```python
from build123d import *

# Parameters (mm, degrees)
SKETCH001_R  = 0.965047
PAD_DEPTH    = 4
SKETCH_W     = 14.86762
SKETCH_H     = 20
PAD001_DEPTH = 5


with BuildPart() as part:
    # Sketch001 → Pad (new body)
    with BuildSketch(Plane.XY):
        with BuildLine():
            ThreePointArc((-5, -17.500002), (0, -22.500002), (5, -17.500002))
            Line((5, -17.500002), (5, 0))
            Line((5, 0), (5, 17.500002))
            ThreePointArc((5, 17.500002), (-2e-06, 22.499991), (-5, 17.499998))
            Line((-5, -17.500002), (-5, 17.499998))
        make_face()
        with Locations((0, 17.499991)):
            Circle(SKETCH001_R, mode=Mode.SUBTRACT)
        with Locations((0, -17.500002)):
            Circle(SKETCH001_R, mode=Mode.SUBTRACT)
    extrude(amount=PAD_DEPTH)

    # Sketch (on Face7 of Pad) → Pad001 (join)
    with BuildSketch(Plane.XY.offset(4)):
        with Locations((0.040686, 0)):
            Rectangle(SKETCH_W, SKETCH_H)
    extrude(amount=-PAD001_DEPTH)


solid = part.part
```
Part model, mm, in its own coordinate system. A direction names the side the tool comes from. Round coordinates to 2 decimals unless told otherwise and drop trailing zeros. Loops run counter-clockwise (first coordinate to the right, second up) from the corner with the lowest first, then second, coordinate; pieces in that order, holes last. Notation, with made-up numbers: (-15.5, 39.25) -> (18.5, 39.25) arc R20 cw to (18.5, 64.25) -> close; hole circle Ø3 at (44, 75). An arc over 180 degrees is marked (long way). Use CSV: the item, a comma, the result in double quotes. Start each with the question number.
1) Cut at A-A, the plane z = 2.8. Write the cut outline in (x, y), plus the area to 3 significant figures.
2) Which spindle directions (+Z, -Z, +X, -X, +Y, -Y) get a long thin tool onto all of the face, cutting with end or side? Do faces 4 (the flat face through (-5, 14, 2)), 5 (the flat face through (5, 14, 2)), 6 (the flat face through (-5, -14, 2)), 7 (the flat face through (5, -14, 2)), 8 (the flat face through (0, 16, 0)). Say none if no direction does.
3) Cut at D-D, the plane x = 2.25. Write the cut outline in (y, z).
4) Cut at B-B, the plane x = 0. Write the cut outline in (y, z).
5) Pull direction Y, two halves, no side cores. Call faces 1 (the cylindrical face through (-0.126, -16.543, 1.972)), 2 (the flat face through (7.474, 0, 2)), 3 (the cylindrical face through (-0.1, -22.5, 2)): +Y half, -Y half, draft (parallel to the pull), parting line (faces both ways), or undercut.
6) Drop flat-ended pins along their axis: P1, Ø1.7, axis at x = 0, y = -17.5, coming from the -Z side; P2, Ø8, axis at x = 1.5, y = 18, coming from the -Z side; P3, Ø1, axis at y = 11.5, z = 3, coming from the +X side; P4, Ø2, axis at x = 2.5, z = 0, coming from the +Y side. Give the stop position or say it passes through.
7) Wall check: L1, parallel to Y at x = 0, z = 1.25; L2, parallel to X at y = -11, z = 1.4; L3, parallel to Z at x = -2.5, y = -11.5. Give the ranges that are in metal, low to high. Write a range as [from, to].
8) Cut at C-C, the plane y = -11.5. Write the cut outline in (x, z).
Determined:
1,outline,"(-7.39, -10) -> (-5, -10) -> (-5, -17.5) arc R5 ccw to (5, -17.5) -> (5, -10) -> (7.47, -10) -> (7.47, 10) -> (5, 10) -> (5, 17.5) arc R5 ccw to (-5, 17.5) -> (-5, 10) -> (-7.39, 10) -> close; hole circle Ø1.93 at (0, -17.5); hole circle Ø1.93 at (0, 17.5)"
1,area,"520 mm2"
2,face 4,"+Z, -Z, -X, +Y"
2,face 5,"+Z, -Z, +X, +Y"
2,face 6,"+Z, -Z, -X, -Y"
2,face 7,"+Z, -Z, +X, -Y"
2,face 8,"-Z, +X, -X, +Y"
3,outline,"(-21.97, 0) -> (-10, 0) -> (-10, -1) -> (10, -1) -> (10, 0) -> (21.97, 0) -> (21.97, 4) -> (-21.97, 4) -> close"
4,outline,"(-22.5, 0) -> (-18.47, 0) -> (-18.47, 4) -> (-22.5, 4) -> close; (-16.53, 0) -> (-10, 0) -> (-10, -1) -> (10, -1) -> (10, 0) -> (16.53, 0) -> (16.53, 4) -> (-16.53, 4) -> close; (18.47, 0) -> (22.5, 0) -> (22.5, 4) -> (18.47, 4) -> close"
5,face 1,"undercut"
5,face 2,"draft"
5,face 3,"-Y half"
6,P1,"passes through"
6,P2,"stops at z = 0"
6,P3,"stops at x = 5"
6,P4,"stops at y = 22.27"
7,L1,"y = [-22.5, -18.47], [-16.53, 16.53], [18.47, 22.5]"
7,L2,"x = [-5, 5]"
7,L3,"z = [0, 4]"
8,outline,"(-5, 0) -> (5, 0) -> (5, 4) -> (-5, 4) -> close"
